from build123d import *

# Parameters (mm, degrees)
F0_W     = 10
F0_H     = 35.0110880776
F0_W_2   = 90
F0_R     = 5
F1_DEPTH = 8
F2_DEPTH = 10
F3_SIZE  = 1
F4_R     = 0.2


with BuildPart() as f1:
    # F0 (on Front) → F1 (new body)
    with BuildSketch(Plane.XZ):
        with Locations((-50, 0)):
            Rectangle(F0_W, F0_H)
        Rectangle(F0_W_2, F0_H)
        with Locations((-35, 0)):
            Circle(F0_R, mode=Mode.SUBTRACT)
        with BuildLine():
            ThreePointArc((-26.5, 0), (-22.5, 4), (-18.5, 0))
            ThreePointArc((-18.5, 0), (-22.5, -4), (-26.5, 0))
        make_face(mode=Mode.SUBTRACT)
        with BuildLine():
            ThreePointArc((26.5, 0), (22.5, -4), (18.5, 0))
            ThreePointArc((18.5, 0), (22.5, 4), (26.5, 0))
        make_face(mode=Mode.SUBTRACT)
        with BuildLine():
            ThreePointArc((40, 0), (35, -5), (30, 0))
            ThreePointArc((30, 0), (35, 5), (40, 0))
        make_face(mode=Mode.SUBTRACT)
        with Locations((50, 0)):
            Rectangle(F0_W, F0_H)
    extrude(amount=-F1_DEPTH)

    # F0 (on Front) → F2 (join)
    with BuildSketch(Plane.XZ):
        Rectangle(F0_W_2, F0_H)
        with Locations((-35, 0)):
            Circle(F0_R, mode=Mode.SUBTRACT)
        with BuildLine():
            ThreePointArc((-26.5, 0), (-22.5, 4), (-18.5, 0))
            ThreePointArc((-18.5, 0), (-22.5, -4), (-26.5, 0))
        make_face(mode=Mode.SUBTRACT)
        with BuildLine():
            ThreePointArc((26.5, 0), (22.5, -4), (18.5, 0))
            ThreePointArc((18.5, 0), (22.5, 4), (26.5, 0))
        make_face(mode=Mode.SUBTRACT)
        with BuildLine():
            ThreePointArc((40, 0), (35, -5), (30, 0))
            ThreePointArc((30, 0), (35, 5), (40, 0))
        make_face(mode=Mode.SUBTRACT)
    extrude(amount=-F2_DEPTH)

    # F3
    f3_edges = [f1.edges().sort_by_distance(p)[0] for p in [
        (55, 4, -17.505544),
        (55, 4, 17.505544),
        (-55, 4, -17.505544),
        (-55, 4, 17.505544),
    ]]
    chamfer(f3_edges, length=F3_SIZE)

    # F4
    f4_edges = [f1.edges().sort_by_distance(p)[0] for p in [
        (45, 8, 0),
        (-45, 8, 0),
    ]]
    fillet(f4_edges, radius=F4_R)


solid = f1.part
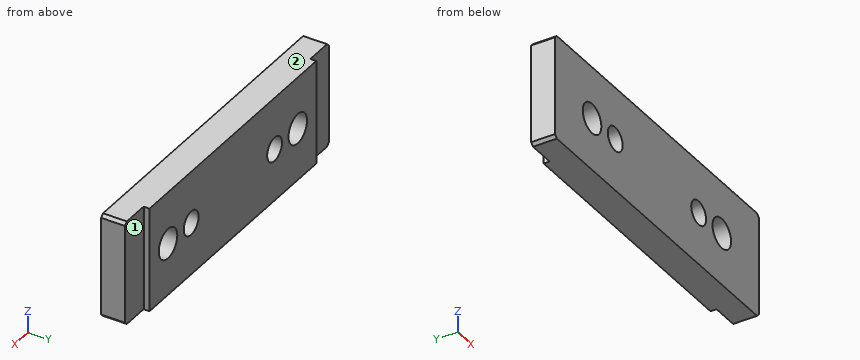
Part model, mm, in its own coordinate system. Face numbers are marked on the shaded views. A direction names the side the tool comes from. Coordinates: 2 decimals unless noted, no trailing zeros. Order: outer loops, then holes, each group sorted by start corner. A loop starts at its lowest first (then second) coordinate and runs counter-clockwise, first axis right, second up. Notation, with made-up numbers: M 58.25,-34 L 77.25,-34 A26 cw 77.25,5 Z; hole C -26.75,24.25 d6. An arc over 180 degrees is marked long. Use a Markdown table: item, result.
(1) Flat gauge pins, fed straight in: pin 1 (7 mm diameter, centred on x = -22.5, z = 0, fed in from +Y); pin 2 (8 mm diameter, centred on x = 51.5, z = 5, fed in from +Y). Where does each tip first touch, or does it go through?
A:
| item | result |
|---|---|
| pin 1 | passes through |
| pin 2 | stops at y = 8 |
(2) Probe L1, parallel to Z at x = -35, y = 5.5; L2, parallel to Y at x = -46, z = -5; L3, parallel to Z at x = -24.5, y = 4.5. List the from-to ranges inside material, lowest first.
A:
| item | result |
|---|---|
| L1 | z = -17.51 to -5, 5 to 17.51 |
| L2 | y = 0 to 8 |
| L3 | z = -17.51 to -3.46, 3.46 to 17.51 |
(3) Cut at A-A on x = -22.5. Write the cut outline in (y, z), then the cut area to 3 significant figures.
A:
| item | result |
|---|---|
| outline | M 0,-17.51 L 10,-17.51 L 10,-4 L 0,-4 Z; M 0,4 L 10,4 L 10,17.51 L 0,17.51 Z |
| area | 270 mm^2 |
(4) Cut at D-D on x = 31. Write the cut outline in (y, z), then the cut area to 3 significant figures.
A:
| item | result |
|---|---|
| outline | M 0,-17.51 L 10,-17.51 L 10,-3 L 0,-3 Z; M 0,3 L 10,3 L 10,17.51 L 0,17.51 Z |
| area | 290 mm^2 |
(5) Cut at B-B on y = 2. Write the cut outline in (x, z).
A:
| item | result |
|---|---|
| outline | M -55,-16.51 L -54,-17.51 L 54,-17.51 L 55,-16.51 L 55,16.51 L 54,17.51 L -54,17.51 L -55,16.51 Z; hole C -35,0 d10; hole C -22.5,0 d8; hole C 22.5,0 d8; hole C 35,0 d10 |
(6) Tool access for the marked faces 1 and 2: list every direction of +Z, -Z, +X, -X, +Y, -Y with a clear straight run to the whole face (end or side of a thin tool).
A:
| item | result |
|---|---|
| face 1 | +Z, -Z, +X, +Y |
| face 2 | +Z, +X, -X, +Y, -Y |
(7) Cut at C-C on z = 0. Write the cut outline in (x, y).
A:
| item | result |
|---|---|
| outline | M -55,0 L -40,0 L -40,10 L -45,10 L -45,8.2 A0.2 cw -45.2,8 L -55,8 Z; M -30,0 L -26.5,0 L -26.5,10 L -30,10 Z; M -18.5,0 L 18.5,0 L 18.5,10 L -18.5,10 Z; M 26.5,0 L 30,0 L 30,10 L 26.5,10 Z; M 40,0 L 55,0 L 55,8 L 45.2,8 A0.2 cw 45,8.2 L 45,10 L 40,10 Z |
